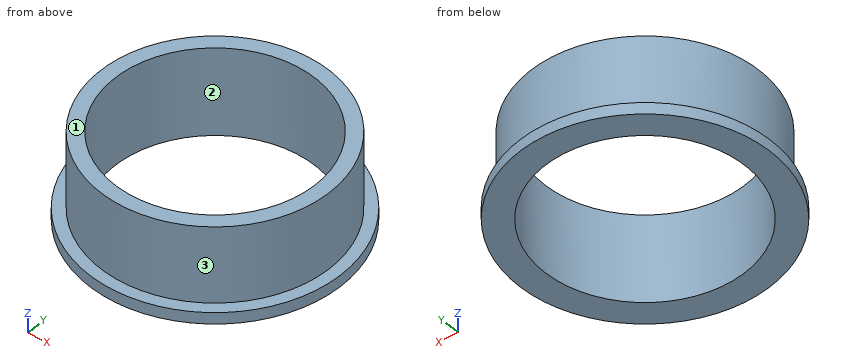
Autodesk Inventor part; units mm, degrees
ref_plane "YZ Plane" through (0, 0, 0) normal (1, 0, 0) x (0, 1, 0)
ref_plane "XZ Plane" through (0, 0, 0) normal (0, 1, 0) x (-1, 0, 0)
ref_plane "XY Plane" through (0, 0, 0) normal (0, 0, 1) x (1, 0, 0)
sketch "Sketch1" plane through (0, 0, 0) normal (0, 0, 1) x (1, 0, 0)
  circle A0 centre (0, 0) radius 8.382
  dimension "d0" = 16.764
extrude "Extrusion1" add sketch "Sketch1" along normal blind 0.762
sketch "Sketch3" plane through (0, 0, 0.762) normal (0, 0, 1) x (1, 0, 0)
  circle A0 centre (0, 0) radius 8.382
  circle A1 centre (0, 0) radius 7.62
  dimension "d13" = 15.24
extrude "Extrusion2" add sketch "Sketch3" along normal blind 5.08 contours A1
sketch "Sketch4" plane through (0, 0, 5.842) normal (0, 0, 1) x (1, 0, 0)
  circle A0 centre (0, 0) radius 7.62
  circle A1 centre (0, 0) radius 6.6675
  dimension "d16" = 13.335
extrude "Extrusion3" cut sketch "Sketch4" against normal through all contours A1
thread "Thread2"
properties part number "base_a"
The listing builds one solid part. Answer for the finished solid, in the listing's coordinates (mm). Face numbers are marked on the shaded views. Coordinates: 2 decimals unless noted, no trailing zeros. Loops run counter-clockwise (first coordinate to the right, second up) from the corner with the lowest first, then second, coordinate; pieces in that order, holes last. Notation, with made-up numbers: (17, -28.5) - (34, -28.5) arc R22 cw to (34, -21.5) - close; hole circle Ø8 at (63, 44.5). An arc over 180 degrees is marked (long way). Write item = value, one per line.
1) Find the intervals of material crossed by line 1 along Y through (x, z) = (0, 2.4); line 2 along X through (y, z) = (-5, 2.05); line 3 along X through (y, z) = (-6, 1), in increasing order.
Responses:
line_1 = -7.62 to -6.67, 6.67 to 7.62
line_2 = -5.75 to -4.41, 4.41 to 5.75
line_3 = -4.7 to -2.91, 2.91 to 4.7
2) Section C-C (z = 3.75) is taken. Determine the outline of the cut face in (x, y) (1 decimal), plus the area to 3 significant figures.
Responses:
outline = circle Ø15.2 at (0, 0); hole circle Ø13.3 at (0, 0)
area = 42.8 mm^2
3) Section A-A (x = 0) is taken. Determine the outline of the cut face in (y, z), plus the area to 3 significant figures.
Responses:
outline = (-8.38, 0) - (-6.67, 0) - (-6.67, 5.84) - (-7.62, 5.84) - (-7.62, 0.76) - (-8.38, 0.76) - close; (6.67, 0) - (8.38, 0) - (8.38, 0.76) - (7.62, 0.76) - (7.62, 5.84) - (6.67, 5.84) - close
area = 12.3 mm^2
4) Determine the mould class of the marked faces 1, 2 and 3 for opening direction X: pulls with the +X half, pulls with the -X half, needs draft (parallel to the pull), parting line crosses it, or undercut.
Responses:
face_1 = needs draft
face_2 = undercut
face_3 = parting line crosses it
